Job drawing, mm, ordinate dimensions from the low corner. One solid piece. A direction names the side the tool comes from. Give positions to 0.01 mm unless a question says otherwise; leave off trailing zeros. Write each loop counter-clockwise with the first axis right and the second up, starting at its lowest first coordinate (ties: lowest second). Pieces come first, ordered by that corner, then holes. Notation, with made-up numbers: M 15,-36 L 56,-36 A13 cw 56,-29 Z; hole C -38,-14.5 d3. An arc over 180 degrees is marked long. Use CSV: the item, a comma, the result in double quotes. Start each with the question number.
Item 1: Pin check, flat tips, straight feed: pin 1 (15 mm diameter, centred on y = 46, z = 56.5, fed in from -X); pin 2 (1 mm diameter, centred on x = 19, z = 8.5, fed in from +Y); pin 3 (12 mm diameter, centred on x = 87.5, y = 19.5, fed in from +Z). Stop position of each tip, or through.
Item 2: Drill centre lines: line 1 (Y direction, x = 89, z = 41) (1 decimal); line 2 (Y direction, x = 7, z = 64.5); line 3 (X direction, y = 57.5, z = 17). Where is each one in solid material? Low to high. Write a range as [from, to].
Item 3: Cut at B-B (y = 41). List the corners of the cut face in (x, z), then the cut area to 3 significant figures.
Item 4: Cut at A-A (z = 62.5). List the corners of the cut face in (x, y), then the cut area to 3 significant figures.
Item 5: Which spindle directions (+Z, -Z, +X, -X, +Y, -Y) get a long thin tool onto all of the face, cutting with end or side? Do the marked faces 4, 5 and 6. Say none if no direction does.
Item 6: Cut at D-D (z = 27). List the corners of the cut face in (x, y), then the cut area to 3 significant figures.
Item 7: Mould opens along Y. For the marked faces 1, 2 and 3 say: released by +Y, released by -Y, zero draft, split by the parting line, or undercut.
Item 8: Cut at C-C (x = 18.5). List the corners of the cut face in (y, z).
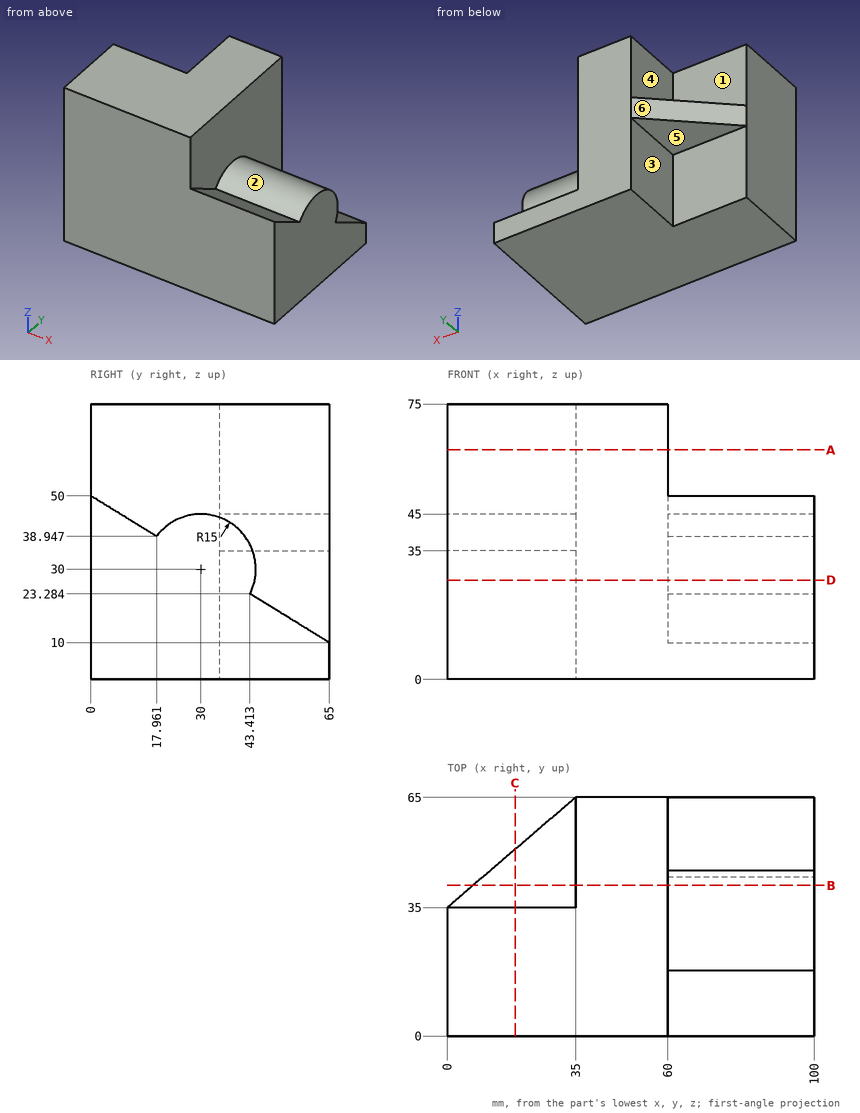
Worked answers:
1,pin 1,"stops at x = 35"
1,pin 2,"stops at y = 35"
1,pin 3,"stops at z = 44.31"
2,line 1,"y = [0, 14.6], [19.8, 40.2]"
2,line 2,"y = [0, 35]"
2,line 3,"x = [35, 60]"
3,outline,"M 7,35 L 35,35 L 35,0 L 100,0 L 100,40.2 L 60,40.2 L 60,75 L 35,75 L 35,45 L 7,45 Z"
3,area,"3,760 mm^2"
4,outline,"M 0,0 L 60,0 L 60,65 L 35,65 L 35,35 L 0,35 Z"
4,area,"2,850 mm^2"
5,face 4,"+Z, -X, +Y"
5,face 5,"-Z, -X, +Y"
5,face 6,"+Z, -Z, -X, +Y"
6,outline,"M 0,0 L 100,0 L 100,44.7 L 60,44.7 L 60,65 L 35,65 L 35,35 L 0,35 Z"
6,area,"4,640 mm^2"
7,face 1,"released by +Y"
7,face 2,"undercut"
7,face 3,"zero draft"
8,outline,"M 0,0 L 35,0 L 35,35 L 50.86,35 L 50.86,45 L 35,45 L 35,75 L 0,75 Z"
